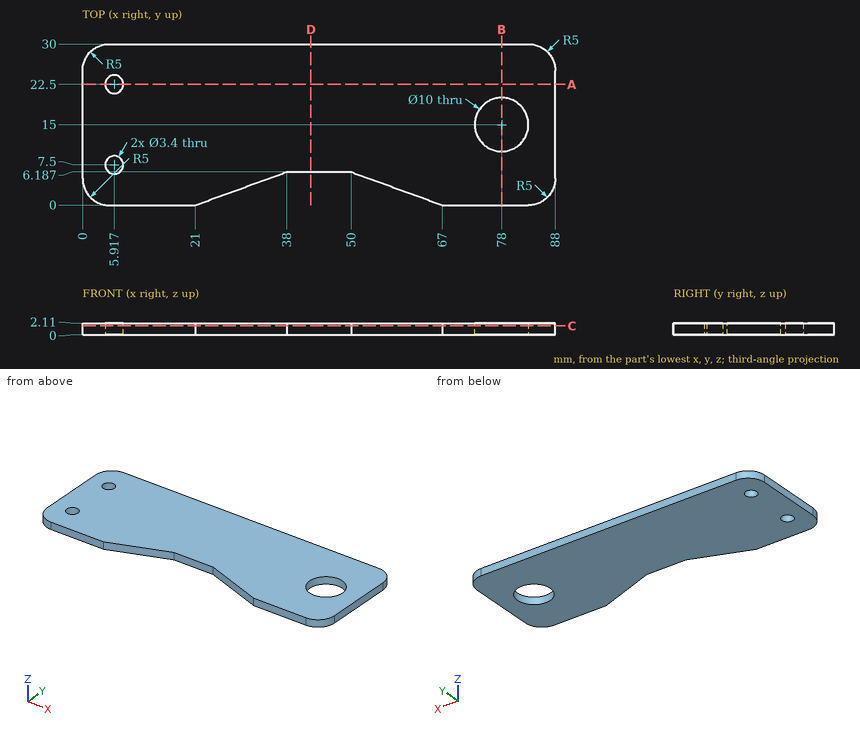
Geometry check sheet. Reference: drawing and pictorial views, mm from the part's lowest x, y, z. Give positions to 0.01 mm unless a question says otherwise; leave off trailing zeros. Write each loop counter-clockwise with the first axis right and the second up, starting at its lowest first coordinate (ties: lowest second). Pieces come first, ordered by that corner, then holes.
Item 1: Cross-section at A-A (y = 22.5). Enter the section's corners in (x, z).
Item 2: Cross-section at B-B (x = 78). Enter the section's corners in (y, z), and give its area (3 significant figures).
Item 3: Scan lines: L1, parallel to Y at x = 78, z = 1.7; L2, parallel to Y at x = 40.5, z = 1.8; L3, parallel to X at y = 15.25, z = 0.6. Record each from-to range of solid material in increasing order.
Item 4: Cross-section at C-C (z = 1.6). Enter the section's corners in (x, y).
Item 5: Gauge pin test, flat ends, axial feed: pin 1 (6 mm diameter, centred on x = 78, y = 15, fed in from -Z); pin 2 (1.1 mm diameter, centred on x = 43, z = 1.5, fed in from -Y). Record the tip position at first contact, or that the pin passes through.
Item 6: Cross-section at D-D (x = 42.5). Enter the section's corners in (y, z).
Report:
1. outline: (0, 0) - (4.22, 0) - (4.22, 2.11) - (0, 2.11) - close; (7.62, 0) - (88, 0) - (88, 2.11) - (7.62, 2.11) - close
2. outline: (0, 0) - (10, 0) - (10, 2.11) - (0, 2.11) - close; (20, 0) - (30, 0) - (30, 2.11) - (20, 2.11) - close
2. area: 42.2 mm2
3. L1: y = 0 to 10, 20 to 30
3. L2: y = 6.19 to 30
3. L3: x = 0 to 73.01, 82.99 to 88
4. outline: (0, 5) arc R5 ccw to (5, 0) - (21, 0) - (38, 6.19) - (50, 6.19) - (67, 0) - (83, 0) arc R5 ccw to (88, 5) - (88, 25) arc R5 ccw to (83, 30) - (5, 30) arc R5 ccw to (0, 25) - close; hole circle Ø3.4 at (5.92, 7.5); hole circle Ø3.4 at (5.92, 22.5); hole circle Ø10 at (78, 15)
5. pin 1: passes through
5. pin 2: stops at y = 6.19
6. outline: (6.19, 0) - (30, 0) - (30, 2.11) - (6.19, 2.11) - close
